Geometry: final body of the model. Coordinates: model frame, mm. Face numbers are marked on the shaded views. A direction names the side the tool comes from. Round coordinates to 2 decimals unless told otherwise and drop trailing zeros. Write each loop counter-clockwise with the first axis right and the second up, starting at its lowest first coordinate (ties: lowest second). Pieces come first, ordered by that corner, then holes.
from build123d import *

# Parameters (mm, degrees)
MOUNT_CYLINDER_DEPTH      = 34.671
MOUNT_CYLINDER_DEPTH_BACK = 34.671
SKETCH1_R                 = 4.5085
SKETCH1_R_2               = 1.9685
SKETCH2_R                 = 5.08
BOSS_EXTRUDE1_DEPTH       = 3.81
BOSS_EXTRUDE3_DEPTH       = 31.75


with BuildPart() as part:
    # Sketch1 → Mount Cylinder (new, two sides: drawn at the far end of the back side and taken through both)
    with BuildSketch(Plane.XY.offset(-MOUNT_CYLINDER_DEPTH_BACK)):
        Circle(SKETCH1_R)
        Circle(SKETCH1_R_2, mode=Mode.SUBTRACT)
    extrude(amount=MOUNT_CYLINDER_DEPTH + MOUNT_CYLINDER_DEPTH_BACK)

    # Sketch2 → Boss-Extrude1 (add)
    with BuildSketch(Plane(origin=(0, 0, 0), x_dir=(1, 0, 0), z_dir=(0, 1, 0))):
        with BuildLine():
            Line((1.9685, -34.671), (6.991111132, -34.671))
            ThreePointArc((6.991111132, -34.671), (13.561283336, -36.502566939), (18.23638307, -41.468978393))
            Line((18.23638307, -41.468978393), (21.83211693, -48.320021607))
            ThreePointArc((21.83211693, -48.320021607), (26.507216664, -53.286433061), (33.077388868, -55.118))
            Line((33.077388868, -55.118), (38.1, -55.118))
            ThreePointArc((38.1, -55.118), (47.080256121, -51.398256121), (50.8, -42.418))
            Line((50.8, -42.418), (50.8, 42.418))
            ThreePointArc((50.8, 42.418), (47.080256121, 51.398256121), (38.1, 55.118))
            Line((38.1, 55.118), (33.077388868, 55.118))
            ThreePointArc((33.077388868, 55.118), (26.507216664, 53.286433061), (21.83211693, 48.320021607))
            Line((21.83211693, 48.320021607), (18.23638307, 41.468978393))
            ThreePointArc((18.23638307, 41.468978393), (13.561283336, 36.502566939), (6.991111132, 34.671))
            Line((6.991111132, 34.671), (1.9685, 34.671))
            Line((1.9685, 34.671), (1.9685, -34.671))
        make_face()
        with Locations(Location((38.1, 42.418, 0), (0, 0, 270))):
            Circle(SKETCH2_R, mode=Mode.SUBTRACT)
        with Locations(Location((38.1, -42.418, 0), (0, 0, 270))):
            Circle(SKETCH2_R, mode=Mode.SUBTRACT)
    extrude(amount=BOSS_EXTRUDE1_DEPTH)

    # Sketch3 → Boss-Extrude3 (add, symmetric)
    with BuildSketch(Plane.XY):
        Polygon((0, -4.5085), (0, -1.9685), (4.056054733, -1.9685), (4.056054733, 0), (50.8, 0), align=None)
    extrude(amount=BOSS_EXTRUDE3_DEPTH, both=True)


solid = part.part
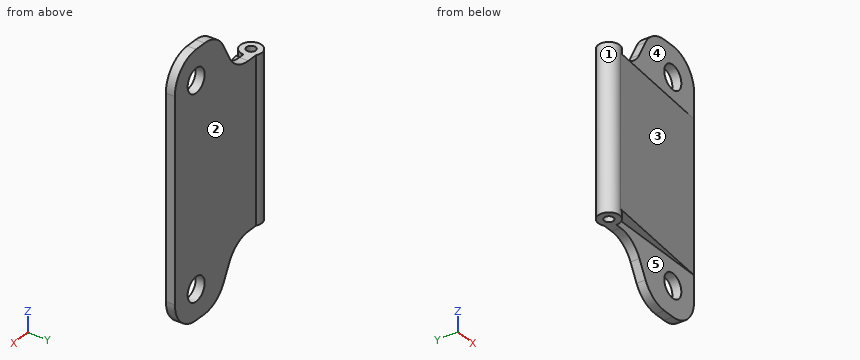
1) Section C-C on x = 25.5. Output: boundary loops of the cut face in (y, z), plus the area to 3 significant figures.
2) Reachability of the marked faces 4 and 5 from +Z, -Z, +X, -X, +Y, -Y: full face, straight path, thin tool, end or side. Return the list, or none.
3) First-contact query: P1, Ø3, axis at x = 7, z = 3.5, coming from the -Y side; P2, Ø6, axis at x = 20.5, z = -30, coming from the +Y side; P3, Ø3, axis at x = 14.5, y = 1, coming from the -Z side. Flat tips, straight axial feed; report the tip coordinate or a pass-through.
4) Line query: probe 1 along Z at (x, y) = (38, 2.5); probe 2 along Z at (x, y) = (33.5, 2.75); probe 3 along X at (y, z) = (0.25, 20.5). Output: solid intervals per line, ascending.
5) Section B-B on x = 11. Output: boundary loops of the cut face in (y, z).
6) Draft query along Y for the marked faces 1, 2 and 3. Return one class per face: pulls with the +Y half, pulls with the -Y half, needs draft (parallel to the pull), parting line crosses it, or undercut.
7) Section A-A on z = 3.5. Output: boundary loops of the cut face in (x, y).
Filled in:
1. outline: (-2.25, -31.75) - (0, -31.75) - (0, -52.61) - (3.81, -52.61) - (3.81, 52.61) - (0, 52.61) - (0, 31.75) - (-2.25, 31.75) - close
1. area: 543 mm2
2. face 4: +Z, +X, -Y
2. face 5: -Z, +X, -Y
3. P1: stops at y = -4.02
3. P2: stops at y = 3.81
3. P3: stops at z = -38.42
4. probe 1: z = -55.12 to -47.5, -37.34 to 37.34, 47.5 to 55.12
4. probe 2: z = -55.12 to -44.57, -40.26 to 40.26, 44.57 to 55.12
4. probe 3: x = -4.5 to -1.95, 1.95 to 50.8
5. outline: (-3.53, -31.75) - (0, -31.75) - (0, -35.32) - (3.81, -35.32) - (3.81, 35.32) - (0, 35.32) - (0, 31.75) - (-3.53, 31.75) - close
6. face 1: parting line crosses it
6. face 2: pulls with the +Y half
6. face 3: pulls with the -Y half
7. outline: (0.79, -4.44) - (50.8, 0) - (50.8, 3.81) - (2.41, 3.81) arc R4.51 ccw (long way) to start; hole circle Ø3.94 at (0, 0)
